Source: CAD feature listing. Evaluate the final solid. Frame: model axes, mm. A direction names the side the tool comes from. Coordinates: 2 decimals unless noted, no trailing zeros. Loops run counter-clockwise (first coordinate to the right, second up) from the corner with the lowest first, then second, coordinate; pieces in that order, holes last. Notation, with made-up numbers: (50.25, 48.5) -> (54.25, 48.5) arc R29 cw to (54.25, 83.5) -> close; hole circle Ø3 at (74, 69). An arc over 180 degrees is marked (long way). Answer as CSV lines item,"result".
from build123d import *

# Parameters (mm, degrees)
BOSS_EXTRUDE1_DEPTH = 48
SKETCH4_R           = 3.15
SKETCH4_R_2         = 2
CUT_EXTRUDE2_DEPTH  = 4.7
SKETCH6_R           = 2.05
BOSS_EXTRUDE3_DEPTH = 9.18
SKETCH4_3_R         = 2
CUT_EXTRUDE3_DEPTH  = 8
FILLET3_R           = 4
FILLET4_R           = 6
BOSS_EXTRUDE4_DEPTH = 48
CUT_EXTRUDE6_START  = -5
SKETCH3_R           = 4.1
CUT_EXTRUDE6_DEPTH  = 66
SKETCH3_3_R         = 2.05
CUT_EXTRUDE7_DEPTH  = 7


with BuildPart() as part:
    # Sketch2 → Boss-Extrude1 (new body)
    with BuildSketch(Plane(origin=(0, 0, 0), x_dir=(1, 0, 0), z_dir=(0, 1, 0))):
        Polygon((0, 0), (0, -15.62924514), (0, -43.62924514), (36.820194138, -43.62924514), (36.820194138, -15.62924514), align=None)
    extrude(amount=BOSS_EXTRUDE1_DEPTH)

    # Sketch4 → Cut-Extrude2 (cut)
    # profile 1 of 8: a face of its own
    with BuildSketch(Plane.XY.offset(43.62924514)):
        with Locations((10.820194138, 40)):
            Circle(SKETCH4_R)
        with Locations((10.820194138, 40)):
            Circle(SKETCH4_R_2, mode=Mode.SUBTRACT)
    # profile 2 of 8: a face of its own
    with BuildSketch(Plane.XY.offset(43.62924514)):
        with Locations((10.820194138, 40)):
            Circle(SKETCH4_R_2)
    # profile 3 of 8: a face of its own
    with BuildSketch(Plane.XY.offset(43.62924514)):
        with Locations((26.820194138, 40)):
            Circle(SKETCH4_R)
        with Locations((26.820194138, 40)):
            Circle(SKETCH4_R_2, mode=Mode.SUBTRACT)
    # profile 4 of 8: a face of its own
    with BuildSketch(Plane.XY.offset(43.62924514)):
        with Locations((26.820194138, 40)):
            Circle(SKETCH4_R_2)
    # profile 5 of 8: a face of its own
    with BuildSketch(Plane.XY.offset(43.62924514)):
        with Locations((26.820194138, 8)):
            Circle(SKETCH4_R)
        with Locations((26.820194138, 8)):
            Circle(SKETCH4_R_2, mode=Mode.SUBTRACT)
    # profile 6 of 8: a face of its own
    with BuildSketch(Plane.XY.offset(43.62924514)):
        with Locations((26.820194138, 8)):
            Circle(SKETCH4_R_2)
    # profile 7 of 8: a face of its own
    with BuildSketch(Plane.XY.offset(43.62924514)):
        with Locations((10.820194138, 8)):
            Circle(SKETCH4_R)
        with Locations((10.820194138, 8)):
            Circle(SKETCH4_R_2, mode=Mode.SUBTRACT)
    # profile 8 of 8: a face of its own
    with BuildSketch(Plane.XY.offset(43.62924514)):
        with Locations((10.820194138, 8)):
            Circle(SKETCH4_R_2)
    extrude(amount=-CUT_EXTRUDE2_DEPTH, mode=Mode.SUBTRACT)

    # Sketch6 → Boss-Extrude3 (add)
    with BuildSketch(Plane.XZ):
        with BuildLine():
            Line((21.555608411, -8.941223432), (36.820194138, 15.62924514))
            Line((36.820194138, 15.62924514), (36.820194138, 43.62924514))
            Line((36.820194138, 43.62924514), (-23.179805862, 43.62924514))
            Line((-23.179805862, 43.62924514), (4.617828, -23.236779181))
            ThreePointArc((4.617828, -23.236779181), (13.54895559, -29.088670071), (22.279280146, -22.941223432))
            Line((22.279280146, -22.941223432), (21.555608411, -8.941223432))
        make_face()
        with Locations(Location((13.39, -19.59, 0), (0, 0, 270))):
            Circle(SKETCH6_R, mode=Mode.SUBTRACT)
    extrude(amount=BOSS_EXTRUDE3_DEPTH)

    # Sketch4<3> → Cut-Extrude3 (cut)
    with BuildSketch(Plane.XY.offset(43.62924514)):
        with Locations((10.820194138, 40)):
            Circle(SKETCH4_3_R)
        with Locations((26.820194138, 40)):
            Circle(SKETCH4_3_R)
        with Locations((26.820194138, 8)):
            Circle(SKETCH4_3_R)
        with Locations((10.820194138, 8)):
            Circle(SKETCH4_3_R)
    extrude(amount=-CUT_EXTRUDE3_DEPTH, mode=Mode.SUBTRACT)

    # Fillet3
    fillet3_edges = [part.edges().sort_by_distance(p)[0] for p in [
        (22.279280146, -4.59, -22.941223432),
    ]]
    fillet(fillet3_edges, radius=FILLET3_R)

    # Fillet4
    fillet4_edges = [part.edges().sort_by_distance(p)[0] for p in [
        (21.555608411, -4.59, -8.941223432),
    ]]
    fillet(fillet4_edges, radius=FILLET4_R)

    # Sketch6<3> → Boss-Extrude4 (add)
    with BuildSketch(Plane.XZ):
        Polygon((-23.179805862, 43.62924514), (0, 0), (0, 43.62924514), align=None)
        Polygon((-4.239616227, -1.930574343), (0, 0), (-23.179805862, 43.62924514), align=None)
    extrude(amount=-BOSS_EXTRUDE4_DEPTH)

    # Sketch3 → Cut-Extrude6 (cut)
    with BuildSketch(Plane(origin=(0, 0, 0), x_dir=(-0.9205048534524429, 0, -0.3907311284892679), z_dir=(0.3907311284892679, 0, -0.9205048534524429)).offset(CUT_EXTRUDE6_START)):
        with Locations((-7, 40)):
            Circle(SKETCH3_R)
        with Locations((-7, 8)):
            Circle(SKETCH3_R)
    extrude(amount=-CUT_EXTRUDE6_DEPTH, mode=Mode.SUBTRACT)

    # Sketch3<3> → Cut-Extrude7 (cut)
    with BuildSketch(Plane(origin=(0, 0, 0), x_dir=(-0.9205048534524429, 0, -0.3907311284892679), z_dir=(0.3907311284892679, 0, -0.9205048534524429))):
        with Locations((-7, 40)):
            Circle(SKETCH3_3_R)
        with Locations((-7, 8)):
            Circle(SKETCH3_3_R)
    extrude(amount=-CUT_EXTRUDE7_DEPTH, mode=Mode.SUBTRACT)


solid = part.part
(1) Pin query (flat end, axial travel): pin 1 Ø2.5 at (x, y) = (26.82, 8) entering from -Z; pin 2 Ø3 at (x, y) = (27.5, 40) entering from +Z; pin 3 Ø10 at (y, z) = (12.5, -2) entering from +X. Return the tip coordinate at first contact, or that it passes through.
Computed values:
pin 1,"z = 10.85"
pin 2,"z = 38.93"
pin 3,"x = 7.07"
(2) Cut plane B-B (z = -19.59). Return the cut outline in (x, y), then the cut area to 3 significant figures.
Computed values:
outline,"(3.1, -9.18) -> (11.34, -9.18) -> (11.34, 0) -> (3.1, 0) -> close; (15.44, -9.18) -> (22.11, -9.18) -> (22.11, 0) -> (15.44, 0) -> close"
area,"137 mm^2"
(3) Cut plane D-D (z = 4). State how many separate pieces and enclosed holes the cut face has, then the cut area to 3 significant figures.
Computed values:
separate pieces,"1"
enclosed holes,"2"
area,"1,080 mm^2"
(4) Material intervals for L1, parallel to Y at x = -5, z = 29; L2, parallel to X at y = 11, z = 12; L3, parallel to Y at x = 15, z = -17.5, sorted ascending. Write a range as [from, to].
Computed values:
L1,"[-9.18, 3.91], [12.09, 35.91], [44.09, 48]"
L2,"[-10.03, -0.53], [5.55, 28.27]"
L3,"[-9.18, 0]"
(5) Access query for faces 1 (the flat face through (29.584, -4.526, 3.982)), 2 (the flat face through (11, 40, 35.629)), 3 (the flat face through (21.945, -4.526, -16.481)). Directions: +Z, -Z, +X, -X, +Y, -Y. A direction counts if a zero-diameter tool reaches every point of the face in a straight line with its end or side. Return the directions, or none.
Computed values:
face 1,"-Z, +X, +Y, -Y"
face 2,"+Z"
face 3,"+X, +Y, -Y"
(6) Draft query along Y for faces 4 (the flat face through (16, 0, -6)), 5 (the flat face through (-2.15, 23.66, -0.98)), 6 (the cylindrical face through (28.73, 8.6, 37.3)). Return one class per face: released by +Y, released by -Y, zero draft, split by the parting line, or undercut.
Computed values:
face 4,"released by +Y"
face 5,"zero draft"
face 6,"undercut"
(7) Cut plane A-A (y = -3). Return the cut outline in (x, z), then the cut area to 3 significant figures.
Computed values:
outline,"(-23.18, 43.63) -> (4.62, -23.24) arc R9.5 ccw to (21.76, -24.09) arc R4 ccw to (22.23, -21.99) -> (21.65, -10.82) arc R6 cw to (22.55, -7.34) -> (36.82, 15.63) -> (36.82, 43.63) -> close; hole circle Ø4.1 at (13.39, -19.59)"
area,"2,740 mm^2"
